Could you check a few things on this model? Use its own coordinates, in mm. A direction names the side the tool comes from. Give positions to 0.01 mm unless a question says otherwise; leave off trailing zeros. Loops run counter-clockwise (first coordinate to the right, second up) from the corner with the lowest first, then second, coordinate; pieces in that order, holes last. Notation, with made-up numbers: (35, 35.5) -> (42, 35.5) arc R36 cw to (42, 72.5) -> close; hole circle Ø6 at (29.5, 88.25). An arc over 180 degrees is marked (long way). Write each question's results on one line, items separated by ' | '. Start each with the question number.
Q1. Will these pins go through, and if not, where does the flat tip stop? P1, Ø7.5, axis at y = 0, z = 6.5, coming from the -X side; P2, Ø2.5, axis at x = -41.5, z = 7.5, coming from the +Y side; P3, Ø12, axis at y = 2, z = 7.5, coming from the +X side.
Q2. If we section it at B-B, the plane y = 3.75: List the corners of the cut face in (x, z) for me, plus the area to 3 significant figures.
Q3. If we section it at C-C, the plane x = -10.5: List the corners of the cut face in (y, z) for me, plus the area to 3 significant figures.
Q4. We'd pull the mould along Z, two halves only. Please class faces 1 (the face through (40, -9, 1)), 2 (the face through (42, -2.5, 11)), 3 (the face through (-1, 0, 25)): released by +Z, released by -Z, zero draft, split by the parting line, or undercut.
Q5. Which directions (+Z, -Z, +X, -X, +Y, -Y) give clear straight access to the entire face, cutting with the end or side of a thin tool? Please do faces 4 (the face through (-44, -9, 1)), 5 (the face through (40, 9, 1)), 6 (the face through (-40, -9, 1)), 7 (the face through (-42, 2.5, 11)).
Q6. If we section it at A-A, the plane z = 7.5: List the corners of the cut face in (x, y) for me.
Q7. If I drill on line 1 along Z through (x, y) = (43, -8.25); line 2 along Z through (x, y) = (36.5, -4.5); line 3 along X through (y, z) = (2.25, 6), over which ranges is the centre line in solid material (lowest first)?
from build123d import *

# Parameters (mm, degrees)
F1_START = 20
F1_DEPTH = 5
F2_DEPTH = 5
F3_R     = 5
F0_W     = 5
F0_H     = 2.5
F4_DEPTH = 25
F0_H_2   = 7.5
F5_DEPTH = 2.5
F6_R     = 1
F7_R     = 2.49999
F8_R     = 2.49999


# Not quite as in the source:
# - a fillet or chamfer is up to 0.001 mm smaller than in the source, because OpenCascade refuses the exact size


with BuildPart() as f1:
    # F0 (on Top) → F1 (new body)
    with BuildSketch(Plane.XY.offset(F1_START)):
        Polygon((56, 0), (56, 12), (-56, 12), (-56, 0), (-44.5, 0), (-44.5, 2.5), (-44.5, 10), (-39.5, 10), (-39.5, 2.5), (-39.5, 0), (-28, 0), (0, 0), (28, 0), (39.5, 0), (39.5, 2.5), (39.5, 10), (44.5, 10), (44.5, 2.5), (44.5, 0), align=None)
        Polygon((56, -12), (56, 0), (44.5, 0), (44.5, -2.5), (44.5, -10), (39.5, -10), (39.5, -2.5), (39.5, 0), (28, 0), (0, 0), (-28, 0), (-39.5, 0), (-39.5, -2.5), (-39.5, -10), (-44.5, -10), (-44.5, -2.5), (-44.5, 0), (-56, 0), (-56, -12), align=None)
    extrude(amount=F1_DEPTH)

    # F2 (add): faces of the model
    f2_faces = [f1.faces().sort_by_distance(p)[0] for p in [
        (39.5, 0, 22.5),
        (-44.5, 0, 22.5),
    ]]
    extrude(f2_faces, amount=F2_DEPTH)

    # F3
    f3_edges = [f1.edges().sort_by_distance(p)[0] for p in [
        (56, -12, 22.5),
        (56, 12, 22.5),
        (-56, -12, 22.5),
        (-56, 12, 22.5),
    ]]
    fillet(f3_edges, radius=F3_R)

    # F0 (on Top) → F4 (join)
    with BuildSketch(Plane.XY):
        with Locations((-42, -1.25)):
            Rectangle(F0_W, F0_H)
        with Locations((-42, 1.25)):
            Rectangle(F0_W, F0_H)
        with Locations((42, 1.25)):
            Rectangle(F0_W, F0_H)
        with Locations((42, -1.25)):
            Rectangle(F0_W, F0_H)
    extrude(amount=F4_DEPTH)

    # F0 (on Top) → F5 (join)
    with BuildSketch(Plane.XY):
        with Locations((-42, -6.25)):
            Rectangle(F0_W, F0_H_2)
        with Locations((-42, 6.25)):
            Rectangle(F0_W, F0_H_2)
        with Locations((42, 6.25)):
            Rectangle(F0_W, F0_H_2)
        with Locations((42, -6.25)):
            Rectangle(F0_W, F0_H_2)
    extrude(amount=F5_DEPTH)

    # F6
    f6_edges = [f1.edges().sort_by_distance(p)[0] for p in [
        (44.5, -2.5, 11.25),
        (39.5, -2.5, 11.25),
        (44.5, 2.5, 11.25),
        (39.5, 2.5, 11.25),
        (-39.5, 2.5, 11.25),
        (-44.5, 2.5, 11.25),
        (-44.5, -2.5, 11.25),
        (-39.5, -2.5, 11.25),
    ]]
    fillet(f6_edges, radius=F6_R)

    # F7 (radius 2.5 in the source; OpenCascade refuses exactly that, so slightly less here)
    f7_edges = [f1.edges().sort_by_distance(p)[0] for p in [
        (-39.5, -10, 1.25),
        (-44.5, -10, 1.25),
        (-39.5, 10, 1.25),
        (-44.5, 10, 1.25),
    ]]
    fillet(f7_edges, radius=F7_R)

    # F8 (radius 2.5 in the source; OpenCascade refuses exactly that, so slightly less here)
    f8_edges = [f1.edges().sort_by_distance(p)[0] for p in [
        (39.5, -10, 1.25),
        (44.5, -10, 1.25),
        (44.5, 10, 1.25),
        (39.5, 10, 1.25),
    ]]
    fillet(f8_edges, radius=F8_R)


solid = f1.part
Final values:
1) P1: stops at x = -44.5 | P2: stops at y = 2.5 | P3: stops at x = 44.5
2) outline: (-56, 20) -> (56, 20) -> (56, 25) -> (-56, 25) -> close; (-44.5, 0) -> (-39.5, 0) -> (-39.5, 2.5) -> (-44.5, 2.5) -> close; (39.5, 0) -> (44.5, 0) -> (44.5, 2.5) -> (39.5, 2.5) -> close | area: 585 mm²
3) outline: (-12, 20) -> (12, 20) -> (12, 25) -> (-12, 25) -> close | area: 120 mm²
4) face 1: zero draft | face 2: undercut | face 3: released by +Z
5) face 4: -Z, -X, -Y | face 5: -Z, +Y | face 6: -Z, -Y | face 7: +X, -X, +Y
6) outline: (-44.5, -1.5) arc R1 ccw to (-43.5, -2.5) -> (-40.5, -2.5) arc R1 ccw to (-39.5, -1.5) -> (-39.5, 1.5) arc R1 ccw to (-40.5, 2.5) -> (-43.5, 2.5) arc R1 ccw to (-44.5, 1.5) -> close; (39.5, -1.5) arc R1 ccw to (40.5, -2.5) -> (43.5, -2.5) arc R1 ccw to (44.5, -1.5) -> (44.5, 1.5) arc R1 ccw to (43.5, 2.5) -> (40.5, 2.5) arc R1 ccw to (39.5, 1.5) -> close
7) line 1: z = 0 to 2.5, 20 to 25 | line 2: z = 20 to 25 | line 3: x = -44.16 to -39.84, 39.84 to 44.16
